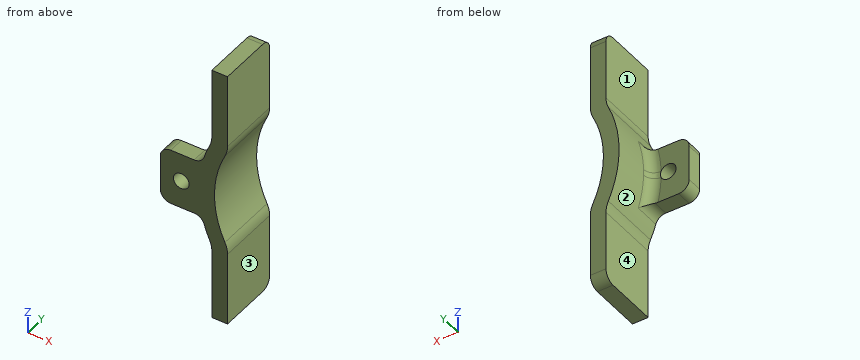
```python
from build123d import *

# Parameters (mm, degrees)
BOSS_EXTRUDE2_DEPTH = 12
FILLET2_R           = 5
FILLET3_R           = 2
SKETCH2_W           = 8
SKETCH2_H           = 10.766845602
SKETCH2_R           = 1.5
BOSS_EXTRUDE3_DEPTH = 3
FILLET4_R           = 2


with BuildPart() as part:
    # Sketch1 → Boss-Extrude2 (new body)
    with BuildSketch(Plane(origin=(0, 0, 0), x_dir=(1, 0, 0), z_dir=(0, 1, 0))):
        with BuildLine():
            Line((-17.5, 25), (-20.5, 25))
            Line((-20.5, 25), (-20.5, 10.428326807))
            ThreePointArc((-20.5, 10.428326807), (-19.132553248, 12.765007099), (-17.5, 14.924811557))
            Line((-17.5, 14.924811557), (-17.5, 25))
        make_face()
        with BuildLine():
            ThreePointArc((-17.5, 14.924811557), (-19.132553248, 12.765007099), (-20.5, 10.428326807))
            Line((-20.5, 10.428326807), (-20.5, -10.428326807))
            ThreePointArc((-20.5, -10.428326807), (-19.132553248, -12.765007099), (-17.5, -14.924811557))
            Line((-17.5, -14.924811557), (-17.5, -9.682458366))
            ThreePointArc((-17.5, -9.682458366), (-20, 0), (-17.5, 9.682458366))
            Line((-17.5, 9.682458366), (-17.5, 14.924811557))
        make_face()
        with BuildLine():
            Line((-20.5, -10.428326807), (-20.5, 10.428326807))
            ThreePointArc((-20.5, 10.428326807), (-23, 0), (-20.5, -10.428326807))
        make_face()
        with BuildLine():
            ThreePointArc((-17.5, -14.924811557), (-19.132553248, -12.765007099), (-20.5, -10.428326807))
            Line((-20.5, -10.428326807), (-20.5, -25))
            Line((-20.5, -25), (-17.5, -25))
            Line((-17.5, -25), (-17.5, -14.924811557))
        make_face()
    extrude(amount=BOSS_EXTRUDE2_DEPTH)

    # Fillet2
    fillet2_edges = [part.edges().sort_by_distance(p)[0] for p in [
        (-17.5, 6, -9.682458366),
        (-17.5, 6, 9.682458366),
        (-20.5, 6, 10.428326807),
        (-20.5, 6, -10.428326807),
    ]]
    fillet(fillet2_edges, radius=FILLET2_R)

    # Fillet3
    fillet3_edges = [part.edges().sort_by_distance(p)[0] for p in [
        (-19, 12, 25),
        (-19, 12, -25),
    ]]
    fillet(fillet3_edges, radius=FILLET3_R)

    # Sketch2 → Boss-Extrude3 (add)
    with BuildSketch(Plane(origin=(0, 0, 0), x_dir=(1, 0, 0), z_dir=(0, 1, 0))):
        with Locations((-26.361099234, 0)):
            Rectangle(SKETCH2_W, SKETCH2_H)
        with Locations(Location((-26.361099234, 0, 0), (0, 0, 270))):
            Circle(SKETCH2_R, mode=Mode.SUBTRACT)
    extrude(amount=BOSS_EXTRUDE3_DEPTH)

    # Fillet4
    fillet4_edges = [part.edges().sort_by_distance(p)[0] for p in [
        (-23, 3, 0),
        (-30.361099234, 1.5, -5.383422801),
        (-30.361099234, 1.5, 5.383422801),
        (-22.361099234, 1.5, 5.383422801),
        (-22.361099234, 1.5, -5.383422801),
    ]]
    fillet(fillet4_edges, radius=FILLET4_R)


solid = part.part
```
Can you work these out from the model? Positions are in its coordinate system, mm. Face numbers are marked on the shaded views. A direction names the side the tool comes from. Give positions to 0.01 mm unless a question says otherwise; leave off trailing zeros. Order: outer loops, then holes, each group sorted by start corner. A loop starts at its lowest first (then second) coordinate and runs counter-clockwise, first axis right, second up. Notation, with made-up numbers: (34.25, -37.75) - (87.25, -37.75) arc R21 cw to (87.25, -13.75) - close; hole circle Ø5 at (36, 87). An arc over 180 degrees is marked (long way). Use a Markdown table: item, result. Add a question column.
Q1. Please list where these lines run through material, in increasing order: line 1 along X through (y, z) = (1.9, 0); line 2 along X through (y, z) = (9.75, 13.5); line 3 along X through (y, z) = (8.5, 0).
Q2. If we section it at D-D on z = -7.5: Write out the boundary of the cut face in (x, y), plus the area to 3 significant figures.
Q3. If we section it at C-C on y = 1.5: Write out the boundary of the cut face in (x, z).
Q4. If we section it at B-B on z = 16.5: Write out the boundary of the cut face in (x, y), plus the area to 3 significant figures.
Q5. If we section it at A-A on y = 6.75: Write out the boundary of the cut face in (x, z), plus the area to 3 significant figures.
Q6. I'm going to push flat-ended pins straight in: pin 1 (4 mm diameter, centred on x = -26.36, z = 0, fed in from +Y); pin 2 (2.5 mm diameter, centred on x = -25, y = 1, fed in from -Z); pin 3 (1.5 mm diameter, centred on x = -26, y = 2, fed in from +Z). Where does each tip first touch, or does it pass through?
Q7. On a 3-axis mill with a long thin cutter (end or side, diameter ignored), from which of +Z, -Z, +X, -X, +Y, -Y can I reach the whole of each face in a straight line? I mean the marked faces 1, 2, 3 and 4. Say none if no direction works.
Answers follow:
| question | item | result |
|---|---|---|
| 1 | line 1 | x = -30.36 to -27.86, -24.86 to -20 |
| 1 | line 2 | x = -20.5 to -17.5 |
| 1 | line 3 | x = -23 to -20 |
| 2 | outline | (-21.74, 0) - (-18.54, 0) - (-18.54, 12) - (-21.74, 12) - close |
| 2 | area | 38.4 mm^2 |
| 3 | outline | (-30.36, -3.38) arc R2 ccw to (-28.36, -5.38) - (-23.88, -5.38) arc R2 cw to (-21.97, -6.79) arc R23 ccw to (-20.95, -9.5) arc R5 cw to (-20.5, -11.57) - (-20.5, -25) - (-17.5, -25) - (-17.5, -10.9) arc R5 ccw to (-18, -8.72) arc R20 cw to (-18, 8.72) arc R5 ccw to (-17.5, 10.9) - (-17.5, 25) - (-20.5, 25) - (-20.5, 11.57) arc R5 cw to (-20.95, 9.5) arc R23 ccw to (-21.97, 6.79) arc R2 cw to (-23.88, 5.38) - (-28.36, 5.38) arc R2 ccw to (-30.36, 3.38) - close; hole circle Ø3 at (-26.36, 0) |
| 4 | outline | (-20.5, 0) - (-17.5, 0) - (-17.5, 12) - (-20.5, 12) - close |
| 4 | area | 36.0 mm^2 |
| 5 | outline | (-20.95, -9.5) arc R5 cw to (-20.5, -11.57) - (-20.5, -25) - (-17.5, -25) - (-17.5, -10.9) arc R5 ccw to (-18, -8.72) arc R20 cw to (-18, 8.72) arc R5 ccw to (-17.5, 10.9) - (-17.5, 25) - (-20.5, 25) - (-20.5, 11.57) arc R5 cw to (-20.95, 9.5) arc R23 ccw to start |
| 5 | area | 152 mm^2 |
| 6 | pin 1 | stops at y = 3.1 |
| 6 | pin 2 | stops at z = -5.39 |
| 6 | pin 3 | stops at z = 5.38 |
| 7 | face 1 | +Z, -X, +Y, -Y |
| 7 | face 2 | -X, +Y |
| 7 | face 3 | +Z, -Z, +X, +Y, -Y |
| 7 | face 4 | -Z, -X, +Y, -Y |
